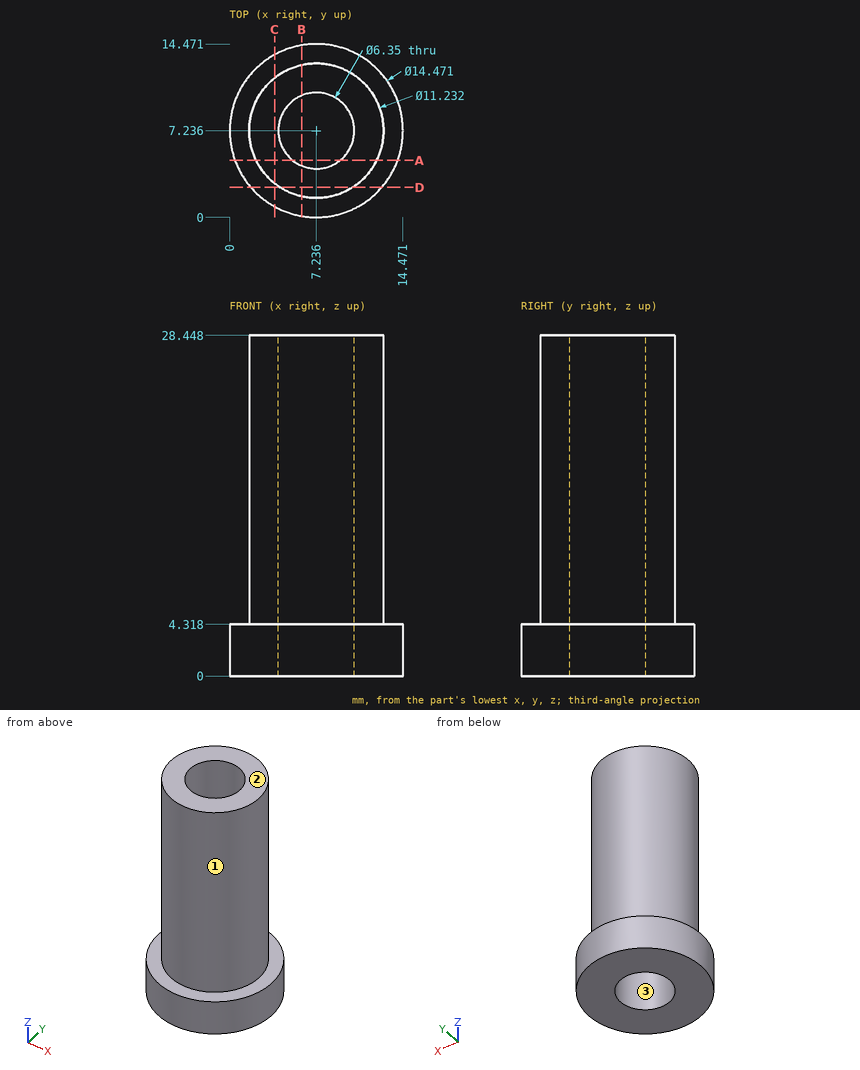
Check sheet for the drawn part. Datum: minimum x, y, z corner. Units: mm. Coordinates: 2 decimals unless noted, no trailing zeros. Loops run counter-clockwise (first coordinate to the right, second up) from the corner with the lowest first, then second, coordinate; pieces in that order, holes last. Notation, with made-up numbers: (-3, -11) -> (39, -11) arc R31 ccw to (39, 14) -> close; hole circle Ø4 at (37.25, -20.75). An arc over 180 degrees is marked (long way). Answer in a Markdown table with one row per item.
1) Draft check along Y on the marked faces 1, 2 and 3. Enter one of: released by +Y, released by -Y, zero draft, split by the parting line, or undercut.
The answers:
| item | result |
|---|---|
| face 1 | split by the parting line |
| face 2 | zero draft |
| face 3 | undercut |
2) Depth check by flat-ended pin: P1, Ø6, axis at x = 12.5, z = 24, coming from the -Y side; P2, Ø1.5, axis at y = 2, z = 25.5, coming from the +X side (1 decimal); P3, Ø3, axis at y = 3.5, z = 25.5, coming from the -X side; P4, Ø1, axis at x = 8, y = 4.5, coming from the +Z side. Enter the tip coordinate at first touch or a pass-through.
The answers:
| item | result |
|---|---|
| P1 | stops at y = 2.1 |
| P2 | stops at x = 10.6 |
| P3 | stops at x = 2.08 |
| P4 | stops at z = 28.45 |
3) Section check C-C (x = 3.75). Record the cut outline in (y, z) (1 decimal), and give its area (3 significant figures).
The answers:
| item | result |
|---|---|
| outline | (0.9, 0) -> (13.6, 0) -> (13.6, 4.3) -> (11.6, 4.3) -> (11.6, 28.4) -> (2.8, 28.4) -> (2.8, 4.3) -> (0.9, 4.3) -> close |
| area | 267 mm2 |
4) Section check A-A (y = 4.75). Record the cut outline in (x, z), and give its area (3 significant figures).
The answers:
| item | result |
|---|---|
| outline | (0.44, 0) -> (5.26, 0) -> (5.26, 28.45) -> (2.2, 28.45) -> (2.2, 4.32) -> (0.44, 4.32) -> close; (9.21, 0) -> (14.03, 0) -> (14.03, 4.32) -> (12.27, 4.32) -> (12.27, 28.45) -> (9.21, 28.45) -> close |
| area | 189 mm2 |
5) Scan lines: line 1 along X through (y, z) = (7.25, 9); line 2 along Z through (x, y) = (4.25, 1.25); line 3 along Y through (x, z) = (6.25, 13.5) (1 decimal). Record each from-to range of solid material in increasing order. Write a range as from..to.
The answers:
| item | result |
|---|---|
| line 1 | x = 1.62..4.06, 10.41..12.85 |
| line 2 | z = 0..4.32 |
| line 3 | y = 1.7..4.2, 10.3..12.8 |
6) Section check D-D (y = 2.5). Record the cut outline in (x, z) (1 decimal), and give its area (3 significant figures).
The answers:
| item | result |
|---|---|
| outline | (1.8, 0) -> (12.7, 0) -> (12.7, 4.3) -> (10.3, 4.3) -> (10.3, 28.4) -> (4.2, 28.4) -> (4.2, 4.3) -> (1.8, 4.3) -> close |
| area | 193 mm2 |
7) Section check B-B (x = 6). Record the cut outline in (y, z) (1 decimal).
The answers:
| item | result |
|---|---|
| outline | (0.1, 0) -> (4.3, 0) -> (4.3, 28.4) -> (1.8, 28.4) -> (1.8, 4.3) -> (0.1, 4.3) -> close; (10.2, 0) -> (14.4, 0) -> (14.4, 4.3) -> (12.7, 4.3) -> (12.7, 28.4) -> (10.2, 28.4) -> close |
